Build history of the part. All positions in model axes, mm. A direction names the side the tool comes from. Round coordinates to 2 decimals unless told otherwise and drop trailing zeros. Loops run counter-clockwise (first coordinate to the right, second up) from the corner with the lowest first, then second, coordinate; pieces in that order, holes last. Notation, with made-up numbers: (37, -7) - (78, -7) arc R15 cw to (78, 14) - close; hole circle Ø10 at (37, 8). An arc over 180 degrees is marked (long way). One line per question, with ' | ' between items. Start each with the question number.
from build123d import *

# Parameters (mm, degrees)
SKETCH_1_W             = 14
SKETCH_1_H             = 4
EXTRUDE_1_DEPTH        = 5
SKETCH_2_W             = 13
SKETCH_2_H             = 3
CUT_EXTRUDE_1_DEPTH    = 3.6
CUT_EXTRUDE_2_REACH    = 17.395
SKETCH_3_W             = 12
SKETCH_3_H             = 3.737461846
SKETCH_4_R             = 0.2
EXTRUDE_2_DEPTH        = 2.75
PATTERN_LINEAR_1_COUNT = 10
PATTERN_LINEAR_1_PITCH = 1.27


with BuildPart() as part:
    # 草图1 → 凸台-拉伸1 (new body)
    with BuildSketch(Plane.XY):
        with Locations((7, 2)):
            Rectangle(SKETCH_1_W, SKETCH_1_H)
    extrude(amount=EXTRUDE_1_DEPTH)

    # 草图2 → 切除-拉伸1 (cut)
    with BuildSketch(Plane.XY.offset(5)):
        with Locations((7, 2)):
            Rectangle(SKETCH_2_W, SKETCH_2_H)
    extrude(amount=-CUT_EXTRUDE_1_DEPTH, mode=Mode.SUBTRACT)

    # 草图3 → 切除-拉伸2 (cut, up to next)
    with BuildSketch(Plane.XZ, mode=Mode.PRIVATE) as cut_extrude_2_sk1:
        with Locations((7, 4.868730923)):
            Rectangle(SKETCH_3_W, SKETCH_3_H)
    cut_extrude_2_tool1 = extrude(cut_extrude_2_sk1.sketch, amount=-CUT_EXTRUDE_2_REACH, mode=Mode.PRIVATE) & part.part
    add(cut_extrude_2_tool1.solids().sort_by_distance((7, 0, 4.868731))[0], mode=Mode.SUBTRACT)

    # 草图4 → 凸台-拉伸2 (add, symmetric)
    with BuildSketch(Plane.XY.offset(1.4)):
        with Locations((1.285, 2.6)):
            Circle(SKETCH_4_R)
    extrude_2 = extrude(amount=EXTRUDE_2_DEPTH, both=True)

    # 阵列(线性)1: 凸台-拉伸2 ×10
    with Locations(*[(i * PATTERN_LINEAR_1_PITCH, 0, 0) for i in range(1, PATTERN_LINEAR_1_COUNT)]):
        add(extrude_2)


solid = part.part
1) Drop flat-ended pins along their axis: pin 1 (2 mm diameter, centred on x = 10.5, y = 0.5, fed in from -Z); pin 2 (1.8 mm diameter, centred on x = 5, z = 3, fed in from -Y); pin 3 (0.6 mm diameter, centred on x = 6, y = 0, fed in from +Z). Give the stop position or say it passes through.
2) Saw through at B-B on x = 12. Write the cut outline in (y, z).
3) Saw through at D-D on y = 3.05. Write the cut outline in (x, z).
4) Saw through at A-A on z = 2.75. State how many separate pieces and enclosed holes the cut face has, and give its area (3 significant figures).
5) Tool access for faces 1 (the flat face through (7, 3.8, 5)), 2 (the flat face through (13.5, 2, 3)): list every direction of +Z, -Z, +X, -X, +Y, -Y with a clear straight run to the whole face (end or side of a thin tool).
6) Wall check: line 1 (X direction, y = 3.15, z = 4.25); line 2 (Z direction, x = 4.5, y = 0.45); line 3 (Z direction, x = 8, y = 0.7). Give the ranges that are in metal, low to high. Write a range as [from, to].
Answer key:
1) pin 1: z = 0 | pin 2: y = 0 | pin 3: z = 3
2) outline: (0, 0) - (4, 0) - (4, 5) - (3.5, 5) - (3.5, 1.4) - (0.5, 1.4) - (0.5, 3) - (0, 3) - close
3) outline: (0, 0) - (14, 0) - (14, 5) - (13.5, 5) - (13.5, 1.4) - (0.5, 1.4) - (0.5, 5) - (0, 5) - close
4) separate pieces: 11 | enclosed holes: 1 | area: 18.3 mm²
5) face 1: +Z, +X, -X, +Y, -Y | face 2: +Z
6) line 1: [0, 0.5], [13.5, 14] | line 2: [0, 3] | line 3: [0, 1.4]
